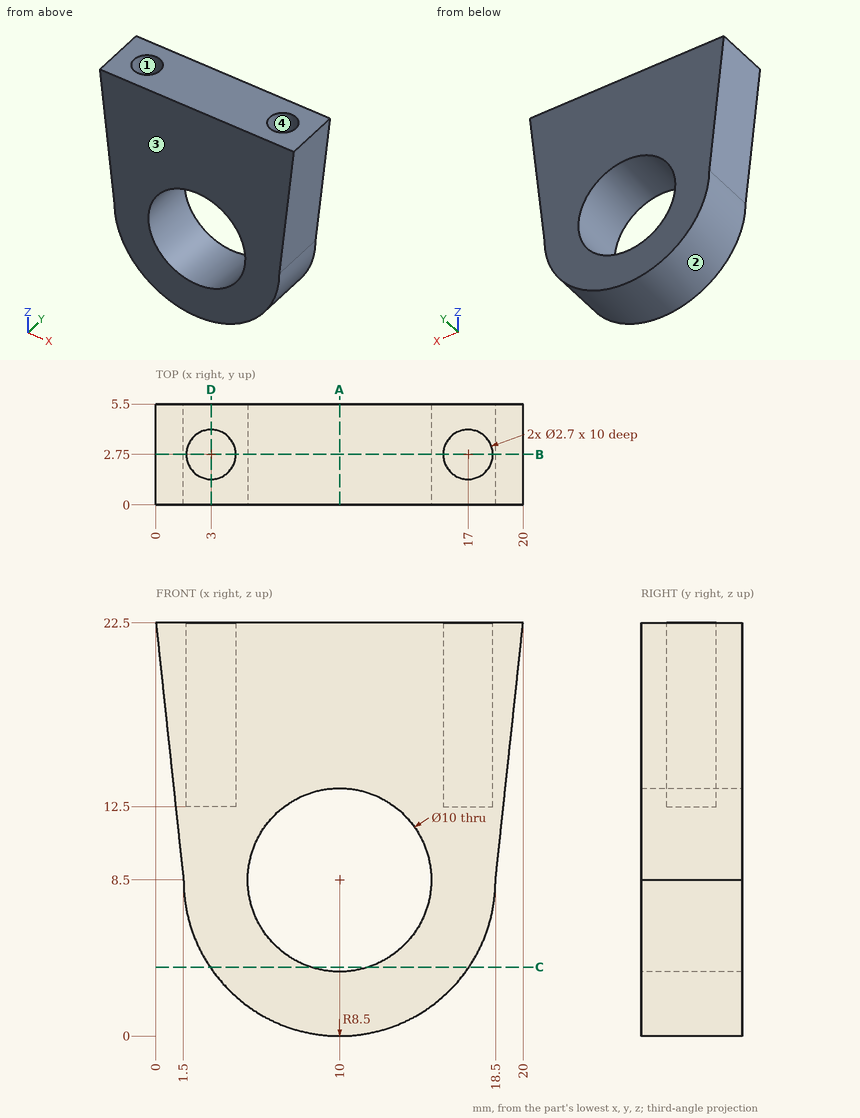
Design review of the part shown in the three views and the two pictorial views. Dimensions are in mm from the part's minimum x, y and z. Give positions to 0.01 mm unless a question says otherwise; leave off trailing zeros. Write each loop counter-clockwise with the first axis right and the second up, starting at its lowest first coordinate (ties: lowest second). Pieces come first, ordered by that corner, then holes.
Item 1: Insertion check: P1, Ø3, axis at y = 2, z = 15, coming from the +X side; P2, Ø2, axis at y = 3, z = 13.5, coming from the +X side; P3, Ø3, axis at x = 3, y = 2.75, coming from the -Z side. Each pin has a flat end and moves straight along its axis. Give the tip position at first contact, or say it passes through.
Item 2: Take a section at D-D (x = 3). Give the boundary of the cut face in (y, z).
Item 3: The part is to be moulded in two halves that separate along Y. For the marked faces 1, 2, 3 and 4, say which applies: +Y half, -Y half, draft (parallel to the pull), parting line (faces both ways), or undercut.
Item 4: Take a section at A-A (x = 10). Give the boundary of the cut face in (y, z).
Item 5: Wall thickness on probe 1 along X at (y, z) = (4.1, 8.5); probe 2 along Z at (x, y) = (10.25, 5.05); probe 3 along Y at (x, z) = (3, 14.75): over which ranges is each line inside the solid? List them lowest first.
Item 6: Take a section at C-C (z = 3.75). Give the boundary of the cut face in (x, y).
Item 7: Take a section at B-B (y = 2.75). Give the boundary of the cut face in (x, z).
Established:
1. P1: stops at x = 19.36
1. P2: stops at x = 19.14
1. P3: stops at z = 2.02
2. outline: (0, 3.68) - (5.5, 3.68) - (5.5, 22.5) - (4.1, 22.5) - (4.1, 12.5) - (1.4, 12.5) - (1.4, 22.5) - (0, 22.5) - close
3. face 1: undercut
3. face 2: draft
3. face 3: -Y half
3. face 4: undercut
4. outline: (0, 0) - (5.5, 0) - (5.5, 3.5) - (0, 3.5) - close; (0, 13.5) - (5.5, 13.5) - (5.5, 22.5) - (0, 22.5) - close
5. probe 1: x = 1.5 to 5, 15 to 18.5
5. probe 2: z = 0 to 3.51, 13.49 to 22.5
5. probe 3: y = 0 to 1.4, 4.1 to 5.5
6. outline: (2.95, 0) - (8.44, 0) - (8.44, 5.5) - (2.95, 5.5) - close; (11.56, 0) - (17.05, 0) - (17.05, 5.5) - (11.56, 5.5) - close
7. outline: (0, 22.5) - (1.5, 8.5) arc R8.5 ccw to (18.5, 8.5) - (20, 22.5) - (18.35, 22.5) - (18.35, 12.5) - (15.65, 12.5) - (15.65, 22.5) - (4.35, 22.5) - (4.35, 12.5) - (1.65, 12.5) - (1.65, 22.5) - close; hole circle Ø10 at (10, 8.5)
